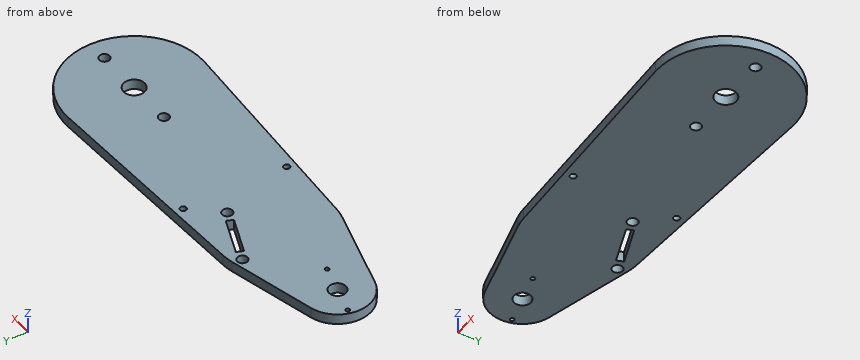
```python
from build123d import *

# Parameters (mm, degrees)
SKETCH1_R           = 16
SKETCH1_R_2         = 4.1
SKETCH1_R_3         = 5.1
BOSS_EXTRUDE1_DEPTH = 5
SKETCH7_R           = 2.5
CUT_EXTRUDE1_DEPTH  = 7
BOSS_EXTRUDE6_DEPTH = 8
SKETCH9_R           = 1.5
CUT_EXTRUDE2_DEPTH  = 6
SKETCH10_R          = 2.5
BOSS_EXTRUDE7_DEPTH = 5
CUT_EXTRUDE4_START  = -10
SKETCH12_R          = 2.5
CUT_EXTRUDE4_DEPTH  = 10
SKETCH11_R          = 1
CUT_EXTRUDE3_DEPTH  = 6
CUT_EXTRUDE5_START  = 5
CUT_EXTRUDE5_DEPTH  = 5


with BuildPart() as part:
    # Sketch1 → Boss-Extrude1 (new body)
    # profile 1 of 3: a face of its own
    with BuildSketch(Plane.XY):
        with BuildLine():
            ThreePointArc((-63.902777778, -26.586845234), (-84.375, 0), (-63.902777778, 26.586845234))
            Line((-63.902777778, 26.586845234), (-105.963888889, 15.468709954))
            ThreePointArc((-105.963888889, 15.468709954), (-92.113397217, 12.677188612), (-85.875, 0))
            ThreePointArc((-85.875, 0), (-92.113397217, -12.677188612), (-105.963888889, -15.468709954))
            Line((-105.963888889, -15.468709954), (-63.902777778, -26.586845234))
        make_face()
    # profile 2 of 3: a face of its own
    with BuildSketch(Plane.XY):
        with Locations((-101.875, 0)):
            Circle(SKETCH1_R)
        with Locations((-101.875, 0)):
            Circle(SKETCH1_R_2, mode=Mode.SUBTRACT)
    # profile 3 of 3: a face of its own
    with BuildSketch(Plane.XY):
        with BuildLine():
            Line((-58.265804598, 27.46480771), (50.206034483, 32.957769253))
            ThreePointArc((50.206034483, 32.957769253), (84.875, 0), (50.206034483, -32.957769253))
            Line((50.206034483, -32.957769253), (-58.265804598, -27.46480771))
            ThreePointArc((-58.265804598, -27.46480771), (-84.375, 0), (-58.265804598, 27.46480771))
        make_face()
        with Locations((51.875, 0)):
            Circle(SKETCH1_R_3, mode=Mode.SUBTRACT)
    extrude(amount=BOSS_EXTRUDE1_DEPTH)

    # Sketch7 → Cut-Extrude1 (cut)
    with BuildSketch(Plane.XY.offset(5)):
        with Locations((29.375, 0)):
            Circle(SKETCH7_R)
        with Locations((74.375, 0)):
            Circle(SKETCH7_R)
    extrude(amount=-CUT_EXTRUDE1_DEPTH, mode=Mode.SUBTRACT)

    # Sketch8 → Boss-Extrude6 (add)
    with BuildSketch(Plane.XY.offset(5)):
        Polygon((-26.375, 28.464101615), (-28.375, 25), (-26.375, 21.535898385), (-22.375, 21.535898385), (-20.375, 25), (-22.375, 28.464101615), align=None)
        Polygon((-25.991580754, 27.8), (-27.608161507, 25), (-25.991580754, 22.2), (-22.758419246, 22.2), (-21.141838493, 25), (-22.758419246, 27.8), align=None, mode=Mode.SUBTRACT)
    boss_extrude6 = extrude(amount=-BOSS_EXTRUDE6_DEPTH)

    # Sketch9 → Cut-Extrude2 (cut)
    with BuildSketch(Plane.XY.offset(5)):
        with Locations((-24.375, 25)):
            Circle(SKETCH9_R)
    cut_extrude2 = extrude(amount=-CUT_EXTRUDE2_DEPTH, mode=Mode.SUBTRACT)

    # Mirror1: Boss-Extrude6 across plane
    add(boss_extrude6.mirror(Plane.ZX))

    # Mirror2: Cut-Extrude2 across plane
    add(cut_extrude2.mirror(Plane.ZX), mode=Mode.SUBTRACT)

    # Sketch10 → Boss-Extrude7 (add)
    with BuildSketch(Plane.XY.offset(5)):
        with Locations((-36.06831441, 11.178241177)):
            Circle(SKETCH10_R)
        with Locations(Location((-64.742423683, 22.173717984, 0), (0, 0, 180))):
            Circle(SKETCH10_R)
        Polygon((-41.60537748, 11.695000918), (-60.279486753, 18.855841852), (-59.205360613, 21.656958243), (-40.53125134, 14.496117309), align=None)
    extrude(amount=BOSS_EXTRUDE7_DEPTH)

    # Sketch12 → Cut-Extrude4 (cut)
    with BuildSketch(Plane.XY.offset(10).offset(CUT_EXTRUDE4_START)):
        with Locations((-36.06831441, 11.178241177)):
            Circle(SKETCH12_R)
        with Locations((-64.742423683, 22.173717984)):
            Circle(SKETCH12_R)
        Polygon((-59.320493296, 21.915307745), (-40.272901838, 14.611249993), (-41.490244797, 11.436651416), (-60.537836255, 18.740709168), align=None)
    extrude(amount=CUT_EXTRUDE4_DEPTH, mode=Mode.SUBTRACT)

    # Sketch11 → Cut-Extrude3 (cut)
    with BuildSketch(Plane.XY.offset(5)):
        with Locations((-88.581577383, -3.513888889)):
            Circle(SKETCH11_R)
        with Locations((-115.168422617, 3.513888889)):
            Circle(SKETCH11_R)
    extrude(amount=-CUT_EXTRUDE3_DEPTH, mode=Mode.SUBTRACT)

    # Sketch13 → Cut-Extrude5 (cut)
    with BuildSketch(Plane(origin=(0, 0, 0), x_dir=(-1, 0, 0), z_dir=(0, 0, -1)).offset(CUT_EXTRUDE5_START)):
        with BuildLine():
            Line((105.963888889, 15.468709954), (63.902777778, 26.586845234))
            ThreePointArc((63.902777778, 26.586845234), (61.107119662, 27.172397082), (58.265804598, 27.46480771))
            Line((58.265804598, 27.46480771), (-50.206034483, 32.957769253))
            ThreePointArc((-50.206034483, 32.957769253), (-84.875, 0), (-50.206034483, -32.957769253))
            Line((-50.206034483, -32.957769253), (58.265804598, -27.46480771))
            ThreePointArc((58.265804598, -27.46480771), (61.107119662, -27.172397082), (63.902777778, -26.586845234))
            Line((63.902777778, -26.586845234), (105.963888889, -15.468709954))
            ThreePointArc((105.963888889, -15.468709954), (117.875, 0), (105.963888889, 15.468709954))
        make_face()
    extrude(amount=-CUT_EXTRUDE5_DEPTH, mode=Mode.SUBTRACT)


solid = part.part
```
Source: CAD feature listing. Evaluate the final solid. Frame: model axes, mm. Coordinates: 2 decimals unless noted, no trailing zeros. Write each loop counter-clockwise with the first axis right and the second up, starting at its lowest first coordinate (ties: lowest second). Pieces come first, ordered by that corner, then holes. Notation, with made-up numbers: (-36, 1.25) -> (-11, 1.25) arc R21 cw to (-11, 19.25) -> close; hole circle Ø4 at (45.5, 25.5). An arc over 180 degrees is marked (long way). Return JSON: item names as keys, results as strings. Group by question number.
1) Contact query for flat-ended pins moving along their axis: P1, Ø2, axis at x = -13.5, z = 4, coming from the -Y side; P2, Ø2, axis at x = 47, z = 2.5, coming from the -Y side; P3, Ø1.5, axis at x = -74, z = 4.5, coming from the -Y side. Output: stop coordinate, or through.
2) Section query C-C, the plane x = -56. Return loops of the section in (y, z), plus the area to 3 significant figures.
3) Section query A-A, the plane y = 0. Return loops of the section in (x, z) (3 decimals), plus the area to 3 significant figures.
4) Ray query, line 1 along Y through (x, z) = (-48.5, 2.35); line 2 along Y through (x, z) = (-56.5, 3.55); line 3 along Y through (x, z) = (-17, 1.5). Return the intervals inside material, ascending.
5) Section query B-B, the plane z = 3.45. State how many separate pieces and enclosed holes the cut face has, plus the area to 3 significant figures.
6) Section query D-D, the plane y = -19. Return loops of the section in (x, z).
From the geometry:
{
 "1": {"P1": "y = -29.78", "P2": "y = -32.85", "P3": "y = -24.12"},
 "2": {"outline": "(-27.58, 0) -> (17, 0) -> (17, 5) -> (-27.58, 5) -> close; (20.64, 0) -> (27.58, 0) -> (27.58, 5) -> (20.64, 5) -> close", "area": "258 mm²"},
 "3": {"outline": "(-117.875, 0) -> (-105.975, 0) -> (-105.975, 5) -> (-117.875, 5) -> close; (-97.775, 0) -> (26.875, 0) -> (26.875, 5) -> (-97.775, 5) -> close; (31.875, 0) -> (46.775, 0) -> (46.775, 5) -> (31.875, 5) -> close; (56.975, 0) -> (71.875, 0) -> (71.875, 5) -> (56.975, 5) -> close; (76.875, 0) -> (84.875, 0) -> (84.875, 5) -> (76.875, 5) -> close", "area": "872 mm²"},
 "4": {"line 1": "-27.96 to 14.12, 17.77 to 27.96", "line 2": "-27.55 to 17.19, 20.83 to 27.55", "line 3": "-29.55 to 29.55"},
 "5": {"separate pieces": "1", "enclosed holes": "11", "area": "10,400 mm²"},
 "6": {"outline": "(-92.6, 0) -> (78.86, 0) -> (78.86, 5) -> (-92.6, 5) -> close"}
}
